Could you check a few things on this model? Use its own coordinates, in mm. A direction names the side the tool comes from. Give positions to 0.01 mm unless a question says otherwise; leave off trailing zeros. Write each loop counter-clockwise with the first axis right and the second up, starting at its lowest first coordinate (ties: lowest second). Pieces come first, ordered by that corner, then holes. Notation, with made-up numbers: (87.5, -18) - (93.5, -18) arc R5 cw to (93.5, -10) - close; hole circle Ø10 at (81, -9). An arc over 180 degrees is marked (long way). Use one line per item in the form item = value.
```python
from build123d import *

# Parameters (mm, degrees)
F1_DEPTH = 50.8


with BuildPart() as f1:
    # F0 (on Top) → F1 (new body)
    with BuildSketch(Plane.XY):
        with BuildLine():
            Line((4.327607, 16.73235), (4.327607, 42.128453))
            Line((4.327607, 42.128453), (-2.022393, 42.128453))
            Line((-2.022393, 42.128453), (-2.022393, 16.728453))
            Line((-2.022393, 16.728453), (-8.366409, 16.728453))
            Line((-8.366409, 16.728453), (-8.366409, -4.005756))
            ThreePointArc((-8.366409, -4.005756), (-6.999831, -7.304968), (-3.700619, -8.671547))
            Line((-3.700619, -8.671547), (17.033591, -8.671547))
            Line((17.033591, -8.671547), (17.033591, -2.26923))
            Line((17.033591, -2.26923), (42.433591, -2.26923))
            Line((42.433591, -2.26923), (42.433591, 4.076364))
            Line((42.433591, 4.076364), (17.033591, 4.076364))
            Line((17.033591, 4.076364), (4.327607, 16.73235))
        make_face()
    extrude(amount=F1_DEPTH)


solid = f1.part
```
1. For pin 1 (10 mm diameter, centred on y = 33, z = 22.5, fed in from +X); pin 2 (4 mm diameter, centred on y = 17, z = 27.5, fed in from +X); pin 3 (12.5 mm diameter, centred on x = 30.5, z = 22.5, fed in from +Y); pin 4 (3 mm diameter, centred on x = 18.5, y = 6.5, fed in from -Z), each with a flat end and sliding along its axis, tell me the tip position at first contact or that it passes through.
Response values:
pin_1 = 4.33
pin_2 = 6.07
pin_3 = 4.08
pin_4 = through
2. Imagine slicing it at C-C, the plane x = 19. List the corners of the cut face in (y, z) for me, and give its area (3 significant figures).
Response values:
outline = (-2.27, 0) - (4.08, 0) - (4.08, 50.8) - (-2.27, 50.8) - close
area = 322 mm²
3. If I drill on line 1 (Y direction, x = 31, z = 17); line 2 (X direction, y = 22, z = 36.5); line 3 (Y direction, x = -4, z = 8), over which ranges is the centre line in solid material (lowest first)? Write a range as from..to.
Response values:
line_1 = -2.27..4.08
line_2 = -2.02..4.33
line_3 = -8.66..16.73
4. Imagine slicing it at A-A, the plane z = 22. List the corners of the cut face in (x, y) for me.
Response values:
outline = (-8.37, -4.01) arc R4.67 ccw to (-3.7, -8.67) - (17.03, -8.67) - (17.03, -2.27) - (42.43, -2.27) - (42.43, 4.08) - (17.03, 4.08) - (4.33, 16.73) - (4.33, 42.13) - (-2.02, 42.13) - (-2.02, 16.73) - (-8.37, 16.73) - close
5. Which directions (+Z, -Z, +X, -X, +Y, -Y) give clear straight access to the entire face, cutting with the end or side of a thin tool? Please do faces 1 (the face through (30, -2.269, 25)), 2 (the face through (30, 4.076, 25)), 3 (the face through (-2.022, 30, 25)).
Response values:
face_1 = +Z, -Z, +X, -Y
face_2 = +Z, -Z, +X, +Y
face_3 = +Z, -Z, -X, +Y
6. Imagine slicing it at B-B, the plane y = 22. List the corners of the cut face in (x, z) for me.
Response values:
outline = (-2.02, 0) - (4.33, 0) - (4.33, 50.8) - (-2.02, 50.8) - close
